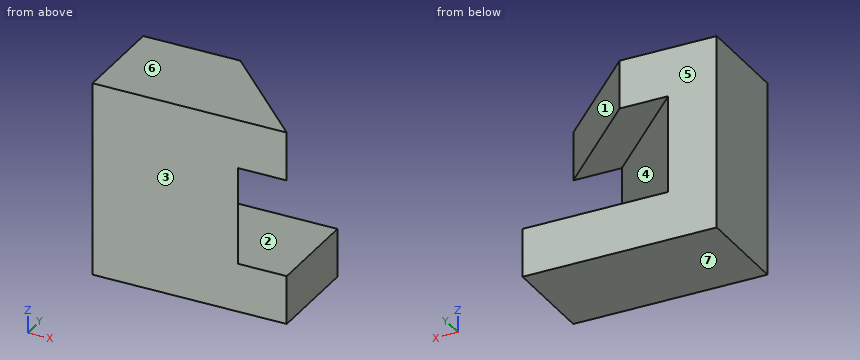
```python
from build123d import *

# Parameters (mm, degrees)
EXTRUDE_1_DEPTH     = 10
CUT_EXTRUDE_START   = -5
CUT_EXTRUDE_1_DEPTH = 10
CUT_EXTRUDE_2_DEPTH = 5


with BuildPart() as part:
    # 草圖1 → 填料-伸長1 (new body)
    with BuildSketch(Plane(origin=(0, 0, 0), x_dir=(1, 0, 0), z_dir=(0, 1, 0))):
        Polygon((10, 5), (10, 10), (-10, 10), (-10, -10), (10, -10), (10, -5), (5, -5), (5, 5), align=None)
    extrude(amount=EXTRUDE_1_DEPTH)

    # 草圖2 → 除料-伸長1 (cut)
    with BuildSketch(Plane.XY.offset(10).offset(CUT_EXTRUDE_START)):
        Polygon((10, 0), (10, 10), (-5, 10), (5, 0), align=None)
    extrude(amount=-CUT_EXTRUDE_1_DEPTH, mode=Mode.SUBTRACT)

    # 草圖3 → 除料-伸長2 (cut)
    with BuildSketch(Plane.XY.offset(10)):
        Polygon((0, 10), (10, 0), (10, 10), align=None)
    extrude(amount=-CUT_EXTRUDE_2_DEPTH, mode=Mode.SUBTRACT)


solid = part.part
```
CAD build for the part. Positions are in the model's coordinates, mm. Face numbers are marked on the shaded views. A direction names the side the tool comes from. Round coordinates to 2 decimals unless told otherwise and drop trailing zeros. Order: outer loops, then holes, each group sorted by start corner. A loop starts at its lowest first (then second) coordinate and runs counter-clockwise, first axis right, second up.
Item 1: Saw through at A-A on x = 6. Write the cut outline in (y, z).
Item 2: Probe line 1 along Z through (x, y) = (3.5, 5); line 2 along Z through (x, y) = (9, 6.75); line 3 along Y through (x, z) = (5, 6.5). List the from-to ranges inside material, lowest first.
Item 3: Saw through at B-B on y = 2.75. Write the cut outline in (x, z).
Item 4: Pin check, flat tip, straight feed: pin 1 (2 mm diameter, centred on x = -4.5, z = -1.5, fed in from +Y). Stop position of the tip, or through.
Item 5: Tool access for the marked faces 1, 2 and 3: list every direction of +Z, -Z, +X, -X, +Y, -Y with a clear straight run to the whole face (end or side of a thin tool).
Item 6: Mould opens along Z. For the marked faces 4, 5, 6 and 7 say: pulls with the +Z half, pulls with the -Z half, needs draft (parallel to the pull), parting line crosses it, or undercut.
Item 7: Saw through at C-C on x = -4.5. Write the cut outline in (y, z), then the cut area to 3 significant figures.
Item 8: Saw through at D-D on z = 5.25. Write the cut outline in (x, y).
Reported:
1. outline: (0, -10) - (10, -10) - (10, -5) - (0, -5) - close; (0, 5) - (4, 5) - (4, 10) - (0, 10) - close
2. line 1: z = -10 to -5, 5 to 10
2. line 2: z = -10 to -5
2. line 3: y = 0 to 5
3. outline: (-10, -10) - (10, -10) - (10, -5) - (2.25, -5) - (2.25, 5) - (7.25, 5) - (7.25, 10) - (-10, 10) - close
4. pin 1: stops at y = 10
5. face 1: +Z, +X, +Y
5. face 2: +X, +Y
5. face 3: +Z, -Z, +X, -X, -Y
6. face 4: undercut
6. face 5: needs draft
6. face 6: pulls with the +Z half
6. face 7: pulls with the -Z half
7. outline: (0, -10) - (10, -10) - (10, -5) - (9.5, -5) - (9.5, 5) - (10, 5) - (10, 10) - (0, 10) - close
7. area: 195 mm2
8. outline: (-10, 0) - (10, 0) - (0, 10) - (-10, 10) - close
